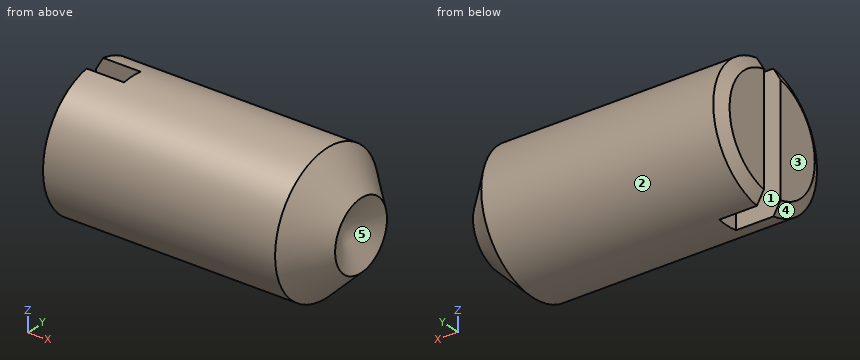
from build123d import *

# Parameters (mm, degrees)
SKETCH2_W  = 5
SKETCH2_H  = 0.8
SLOT_DEPTH = 1.63


with BuildPart() as part:
    # BodySke → BaseBody (revolve)
    with BuildSketch(Plane.XY):
        Polygon((10, 1.25), (9.278312164, 0), (0, 0), (0, 2.055), (0.25692087, 2.5), (8.75, 2.5), align=None)
    revolve(axis=Axis((-12.7, 0, 0), (1, 0, 0)))

    # Sketch2 → Slot (cut)
    with BuildSketch(Plane(origin=(0, 0, 0), x_dir=(0, 0, -1), z_dir=(1, 0, 0))):
        Rectangle(SKETCH2_W, SKETCH2_H)
    extrude(amount=SLOT_DEPTH, mode=Mode.SUBTRACT)


solid = part.part
Design review of the part built by this model. Coordinates are the model's own, in mm. Face numbers are marked on the shaded views. A direction names the side the tool comes from. Round coordinates to 2 decimals unless told otherwise and drop trailing zeros. Order: outer loops, then holes, each group sorted by start corner. A loop starts at its lowest first (then second) coordinate and runs counter-clockwise, first axis right, second up. Notation, with made-up numbers: M -19,16 L 10,16 A23 ccw 10,30 Z; hole C 82,-39 d7. An arc over 180 degrees is marked long. Answer as CSV lines item,"result". Start each with the question number.
1) Tool access review of the marked faces 1 and 2: name each direction out of +Z, -Z, +X, -X, +Y, -Y from which nothing blocks a thin tool from reaching the whole face with its end or side.
2) Wall thickness on line 1 along Y through (x, z) = (3.5, -0.1); line 2 along Y through (x, z) = (9.25, -0.9); line 3 along Z through (x, y) = (4.75, 2.2): over which ranges is each line inside the solid? List them lowest first. Write a range as [from, to].
3) For pin 1 Ø2 at (x, z) = (1.5, -2) entering from -Y; pin 2 Ø1.5 at (x, z) = (6.5, -2) entering from -Y; pin 3 Ø2 at (x, z) = (5, 1.5) entering from -Y, all flat-tipped, find the tip position at first contact; note any pin that passes through.
4) Add section A-A (x = 2.25). Give the boundary of the cut face in (y, z).
5) The part is to be moulded in two halves that separate along Z. For the marked faces 3, 4 and 5, say which applies: +Z half, -Z half, draft (parallel to the pull), parting line (faces both ways), or undercut.
Resolved:
1,face 1,"+Z, -Z, -X"
1,face 2,"+X, -X"
2,line 1,"[-2.5, 2.5]"
2,line 2,"[-1.79, 1.79]"
2,line 3,"[-1.19, 1.19]"
3,pin 1,"y = -2.29"
3,pin 2,"y = -2.17"
3,pin 3,"y = -2.45"
4,outline,"C 0,0 d5"
5,face 3,"draft"
5,face 4,"parting line"
5,face 5,"undercut"
